Autodesk Inventor part; units mm, degrees
ref_plane "YZ Plane" through (0, 0, 0) normal (1, 0, 0) x (0, 1, 0)
ref_plane "XZ Plane" through (0, 0, 0) normal (0, 1, 0) x (-1, 0, 0)
ref_plane "XY Plane" through (0, 0, 0) normal (0, 0, 1) x (1, 0, 0)
sketch "Sketch1" plane through (0, 0, 0) normal (0, 0, 1) x (1, 0, 0)
  line L0 (-59.7338, 79.3295) -> (-59.7338, -47.6705)
  line L1 (-59.7338, -47.6705) -> (67.2662, -47.6705)
  line L2 (67.2662, -47.6705) -> (67.2662, 60.2795)
  line L3 (67.2662, 60.2795) -> (13.2912, 60.2795)
  line L4 (13.2912, 60.2795) -> (13.2912, 15.8295)
  line L5 (13.2912, 15.8295) -> (-8.9338, 15.8295)
  line L6 (-8.9338, 15.8295) -> (-8.9338, 79.3295)
  line L7 (-8.9338, 79.3295) -> (-59.7338, 79.3295)
  line L8 (67.2662, 60.2795) -> (105.3662, 60.2795)
  line L9 (105.3662, 60.2795) -> (105.3662, -47.6705)
  line L10 (105.3662, -47.6705) -> (67.2662, -47.6705)
  point P0 (0, 0)
  point P1 (-47.0338, 66.6295)
  point P2 (54.5662, 47.5795)
  point P3 (41.8662, -3.2205)
  point P4 (54.5662, -34.9705)
  point P5 (-47.0338, -9.5705)
  point P6 (89.4658, -31.7955)
  point P7 (89.4658, -11.8057)
  point P8 (-21.6338, 66.6295)
  point P9 (-21.6338, -9.5705)
  point P10 (29.1662, 47.5795)
  point P11 (54.5662, -34.9705)
  point P12 (54.5662, -9.5705)
  point P13 (29.1662, -34.9705)
  point P14 (89.4658, 44.4045)
  point P15 (89.4658, 24.4147)
  dimension "d0" = 127
  dimension "d1" = 127
  dimension "d2" = 50.8
  dimension "d3" = 53.975
  dimension "d4" = 107.95
  dimension "d5" = 63.5
  dimension "d6" = 12.7
  dimension "d7" = 12.7
  dimension "d8" = 12.7
  dimension "d9" = 12.7
  dimension "d10" = 44.45
  dimension "d11" = 25.4
  dimension "d21" = 12.7
  dimension "d22" = 12.7
  dimension "d23" = 12.7
  dimension "d24" = 38.1
  dimension "d25" = 38.1
  dimension "d26" = 107.95
  dimension "d27" = 15.875
  dimension "d28" = 19.9898
  dimension "d38" = 15.9004
  dimension "d39" = 15.9004
  dimension "d40" = 12.7
  dimension "d41" = 12.7
  dimension "d42" = 25.4
  dimension "d43" = 76.2
  dimension "d44" = 12.7
  dimension "d46" = 12.7
  dimension "d47" = 25.4
  dimension "d48" = 38.1
  dimension "d49" = 12.7
  dimension "d50" = 12.7
  dimension "d51" = 38.1
  dimension "d52" = 25.4
  dimension "d54" = 15.875
  dimension "d55" = 19.9898
  dimension "d56" = 15.9004
  dimension "d57" = 15.9004
extrude "Extrusion1" add sketch "Sketch1" against normal blind 3.175 contours L7 L6 L5 L4 L3 L2 L1 L0
hole "Hole1" at (-47.0338, 66.6295, 0) at (54.5662, 47.5795, 0) at (41.8662, -3.2205, 0) at (-47.0338, -9.5705, 0) at (54.5662, -34.9705, 0) at (89.4658, -31.7955, 0) at (89.4658, -11.8057, 0) at (-21.6338, 66.6295, 0) at (-21.6338, -9.5705, 0) at (29.1662, 47.5795, 0) at (29.1662, -34.9705, 0) direction (0, 0, -1) diameter 6.35 depth 25.4 tip angle 118
extrude "Extrusion2" add sketch "Sketch1" against normal blind 3.175 contours L2 L8 L9 L10
hole "Hole2" at (89.4658, -11.8057, 0) at (89.4658, -31.7955, 0) at (89.4658, 24.4147, 0) at (89.4658, 44.4045, 0) direction (0, 0, -1) diameter 6.35 depth 25.4 tip angle 118
properties part number "AS5-8-5-002"
Verification items for the finished model (mm, model axes). A direction names the side the tool comes from. Coordinates: 2 decimals unless noted, no trailing zeros. Write each loop counter-clockwise with the first axis right and the second up, starting at its lowest first coordinate (ties: lowest second). Pieces come first, ordered by that corner, then holes. Notation, with made-up numbers: (3.25, 85.25) - (10.25, 85.25) arc R9 cw to (10.25, 100.25) - close; hole circle Ø1 at (11.25, -11). An arc over 180 degrees is marked (long way). Answer as a JSON object with one key per item and string values.
(1) Thickness scan on line 1 along X through (y, z) = (48, -0.5); line 2 along X through (y, z) = (55.5, -0.3); line 3 along Y through (x, z) = (-45, -1.95). Record the ranges inside material, lowest first.
Report:
{"line 1": "-59.73 to -8.93, 13.29 to 26.02, 32.31 to 51.42, 57.71 to 105.37", "line 2": "-59.73 to -8.93, 13.29 to 105.37", "line 3": "-47.67 to -12.01, -7.13 to 64.19, 69.07 to 79.33"}
(2) Gauge pin test, flat end, axial feed: pin 1 Ø1 at (x, z) = (55.5, -2.5) entering from +Y. Record the tip position at first contact, or that the pin passes through.
Report:
{"pin 1": "y = 60.28"}
(3) Tool access check on faces 1 (the flat face through (13.291, 38, -2)), 2 (the flat face through (59, 60.28, -2)), 3 (the flat face through (-59.734, 17, -2)). Record the directions out of +Z, -Z, +X, -X, +Y, -Y that give a thin tool (end or side, any length) a straight path to the whole face; none if there is none.
Report:
{"face 1": "+Z, -Z, +Y", "face 2": "+Z, -Z, +X, +Y", "face 3": "+Z, -Z, -X, +Y, -Y"}
(4) Cross-section at C-C on y = -3.5. Record the cut outline in (x, z) (3 decimals).
Report:
{"outline": "(-59.734, -3.175) - (38.704, -3.175) - (38.704, 0) - (-59.734, 0) - close; (45.029, -3.175) - (105.366, -3.175) - (105.366, 0) - (45.029, 0) - close"}
(5) Mould release check, pull along Y, two halves, no side actions. Record for faces 4 (the flat face through (22, 17, 0)), 5 (the flat face through (24, -47.67, -2)), 6 (the cylindrical face through (86.789, -13.513, -1.61)): pulls with the +Y half, pulls with the -Y half, needs draft (parallel to the pull), parting line crosses it, or undercut.
Report:
{"face 4": "needs draft", "face 5": "pulls with the -Y half", "face 6": "undercut"}
(6) Cross-section at B-B on z = -0.8. Give the number of separate pieces and of enclosed holes in the cut face, plus the area to 3 significant figures.
Report:
{"separate pieces": "1", "enclosed holes": "13", "area": "17,400 mm^2"}
(7) Cross-section at A-A on y = 34.5. Record the cut outline in (x, z) (3 decimals).
Report:
{"outline": "(-59.734, -3.175) - (-8.934, -3.175) - (-8.934, 0) - (-59.734, 0) - close; (13.291, -3.175) - (105.366, -3.175) - (105.366, 0) - (13.291, 0) - close"}
